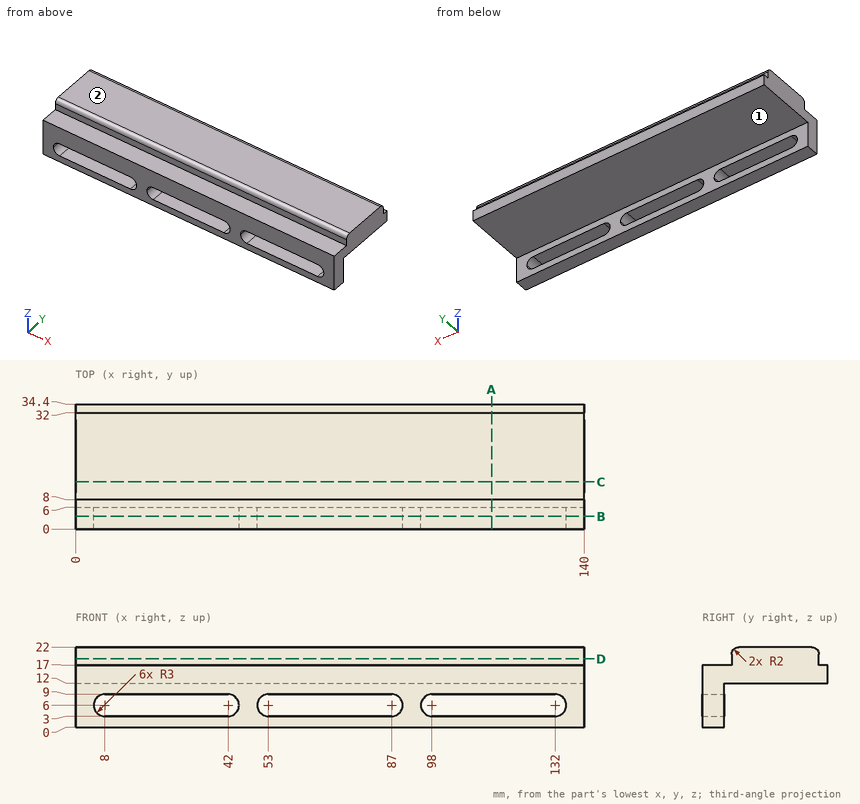
Input: dimensioned drawing with shaded views. Units: mm. Origin: part minimum x, y, z. A direction names the side the tool comes from. Round coordinates to 2 decimals unless told otherwise and drop trailing zeros. Order: outer loops, then holes, each group sorted by start corner. A loop starts at its lowest first (then second) coordinate and runs counter-clockwise, first axis right, second up. Notation, with made-up numbers: (57, 10.5) -> (103, 10.5) arc R17 cw to (103, 38.5) -> close; hole circle Ø9 at (66.5, 40). An arc over 180 degrees is marked (long way). One line per item, written item: value. Start each with the question number.
Q1. Section query C-C (y = 13). Return the cut outline in (x, z).
Q2. Access query for the marked faces 1 and 2. Directions: +Z, -Z, +X, -X, +Y, -Y. A direction counts if a zero-diameter tool reaches every point of the face in a straight line with its end or side. Return the directions, or none.
Q3. Section query A-A (x = 114.5). Return the cut outline in (y, z).
Q4. Material intervals for probe 1 along X at (y, z) = (3, 6); probe 2 along Z at (x, y) = (101, 4.5); probe 3 along Y at (x, z) = (128.5, 2), sorted ascending.
Q5. Section query B-B (y = 3.5). Return the cut outline in (x, z), plus the area to 3 significant figures.
Q6. Pin query (flat end, axial travel): pin 1 (0.7 mm diameter, centred on x = 52, y = 32.5, fed in from +Z); pin 2 (2 mm diameter, centred on x = 26.5, z = 2.5, fed in from -Y); pin 3 (1.5 mm diameter, centred on x = 43.5, z = 18.5, fed in from +Y); pin 4 (0.9 mm diameter, centred on x = 63.5, z = 18, fed in from -Y). Return the tip coordinate at first contact, or that it passes through.
Q7. Section query D-D (z = 18.75). Return the cut outline in (x, y), plus the area to 3 significant figures.
Findings below:
1. outline: (0, 12) -> (140, 12) -> (140, 22) -> (0, 22) -> close
2. face 1: -Z, +X, -X, +Y
2. face 2: +Z, +X, -X, +Y, -Y
3. outline: (0, 0) -> (6, 0) -> (6, 3) -> (0, 3) -> close; (0, 9) -> (6, 9) -> (6, 12) -> (34.4, 12) -> (34.4, 17) -> (32, 17) -> (32, 20) arc R2 ccw to (30, 22) -> (10, 22) arc R2 ccw to (8, 20) -> (8, 17) -> (0, 17) -> close
4. probe 1: 0 to 5, 45 to 50, 90 to 95, 135 to 140
4. probe 2: 0 to 3, 9 to 17
4. probe 3: 0 to 6
5. outline: (0, 0) -> (140, 0) -> (140, 17) -> (0, 17) -> close; hole (5, 6) arc R3 ccw to (8, 3) -> (42, 3) arc R3 ccw to (45, 6) arc R3 ccw to (42, 9) -> (8, 9) arc R3 ccw to start; hole (50, 6) arc R3 ccw to (53, 3) -> (87, 3) arc R3 ccw to (90, 6) arc R3 ccw to (87, 9) -> (53, 9) arc R3 ccw to start; hole (95, 6) arc R3 ccw to (98, 3) -> (132, 3) arc R3 ccw to (135, 6) arc R3 ccw to (132, 9) -> (98, 9) arc R3 ccw to start
5. area: 1,680 mm²
6. pin 1: z = 17
6. pin 2: y = 0
6. pin 3: y = 32
6. pin 4: y = 8
7. outline: (0, 8) -> (140, 8) -> (140, 32) -> (0, 32) -> close
7. area: 3,360 mm²
